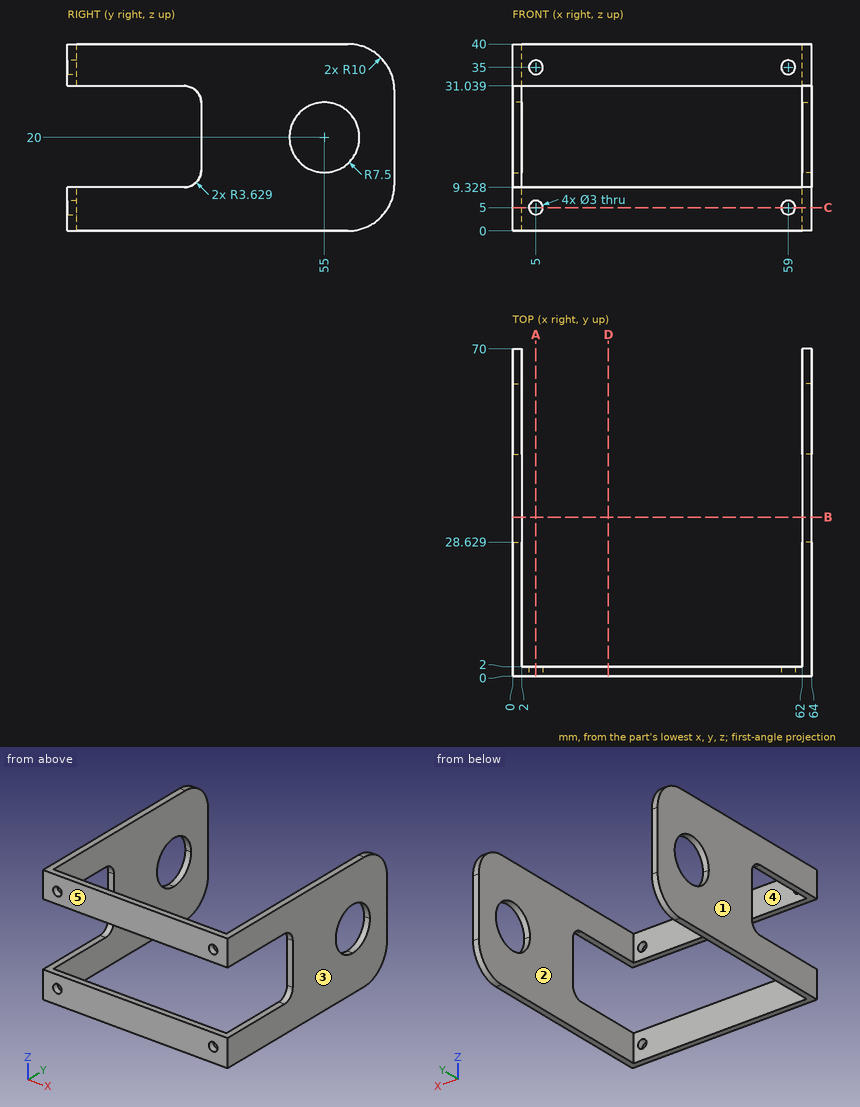
Here's the drawing with two shaded views (mm, measured from the low corner). I have some questions. A direction names the side the tool comes from. Coordinates: 2 decimals unless noted, no trailing zeros. Write each loop counter-clockwise with the first axis right and the second up, starting at its lowest first coordinate (ties: lowest second). Pieces come first, ordered by that corner, then holes. Notation, with made-up numbers: (-9, 41.25) -> (2, 41.25) arc R13 cw to (2, 55.25) -> close; hole circle Ø11 at (44.5, -2). An arc over 180 degrees is marked (long way). Use a Markdown table: item, result. Add a question column.
(1) If we section it at A-A, the plane x = 5: Write out the boundary of the cut face in (y, z).
(2) If we section it at C-C, the plane z = 5: Write out the boundary of the cut face in (x, y).
(3) If we section it at D-D, the plane x = 20.5: Write out the boundary of the cut face in (y, z).
(4) If we section it at B-B, the plane y = 34: Write out the boundary of the cut face in (x, z), and give its area (3 significant figures).
(5) We'd pull the mould along X, two halves only. Please class the marked faces 3, 4 and 5: +X half, -X half, draft (parallel to the pull), parting line (faces both ways), or undercut.
(6) I'm going to push flat-ended pins straight in: P1, Ø1.6, axis at x = 63, z = 17, coming from the -Y side; P2, Ø4.5, axis at x = 39.5, z = 35, coming from the +Y side; P3, Ø1.8, axis at x = 5, z = 35, coming from the +Y side. Where does each tip first touch, or does it pass through?
(7) For the marked faces 1 and 2, which set-ups out of +Z, -Z, +X, -X, +Y, -Y let a thin tool reach every point of the face, with its end or its side?
(8) Please list where these lines run through material, in increasing order: line 1 (Z direction, x = 59, y = 0.55); line 2 (X direction, y = 1.1, z = 5); line 3 (X direction, y = 46, z = 25.5).
Outcome:
| question | item | result |
|---|---|---|
| 1 | outline | (0, 0) -> (2, 0) -> (2, 3.5) -> (0, 3.5) -> close; (0, 6.5) -> (2, 6.5) -> (2, 9.33) -> (0, 9.33) -> close; (0, 31.04) -> (2, 31.04) -> (2, 33.5) -> (0, 33.5) -> close; (0, 36.5) -> (2, 36.5) -> (2, 40) -> (0, 40) -> close |
| 2 | outline | (0, 0) -> (3.5, 0) -> (3.5, 2) -> (2, 2) -> (2, 68.66) -> (0, 68.66) -> close; (6.5, 0) -> (57.5, 0) -> (57.5, 2) -> (6.5, 2) -> close; (60.5, 0) -> (64, 0) -> (64, 68.66) -> (62, 68.66) -> (62, 2) -> (60.5, 2) -> close |
| 3 | outline | (0, 0) -> (2, 0) -> (2, 9.33) -> (0, 9.33) -> close; (0, 31.04) -> (2, 31.04) -> (2, 40) -> (0, 40) -> close |
| 4 | outline | (0, 0) -> (2, 0) -> (2, 40) -> (0, 40) -> close; (62, 0) -> (64, 0) -> (64, 40) -> (62, 40) -> close |
| 4 | area | 160 mm^2 |
| 5 | face 3 | +X half |
| 5 | face 4 | undercut |
| 5 | face 5 | draft |
| 6 | P1 | stops at y = 28.63 |
| 6 | P2 | stops at y = 2 |
| 6 | P3 | passes through |
| 7 | face 1 | +Z, -Z, -X, +Y, -Y |
| 7 | face 2 | +Z, -Z, +Y |
| 8 | line 1 | z = 0 to 3.5, 6.5 to 9.33, 31.04 to 33.5, 36.5 to 40 |
| 8 | line 2 | x = 0 to 3.5, 6.5 to 57.5, 60.5 to 64 |
| 8 | line 3 | x = 0 to 2, 62 to 64 |
